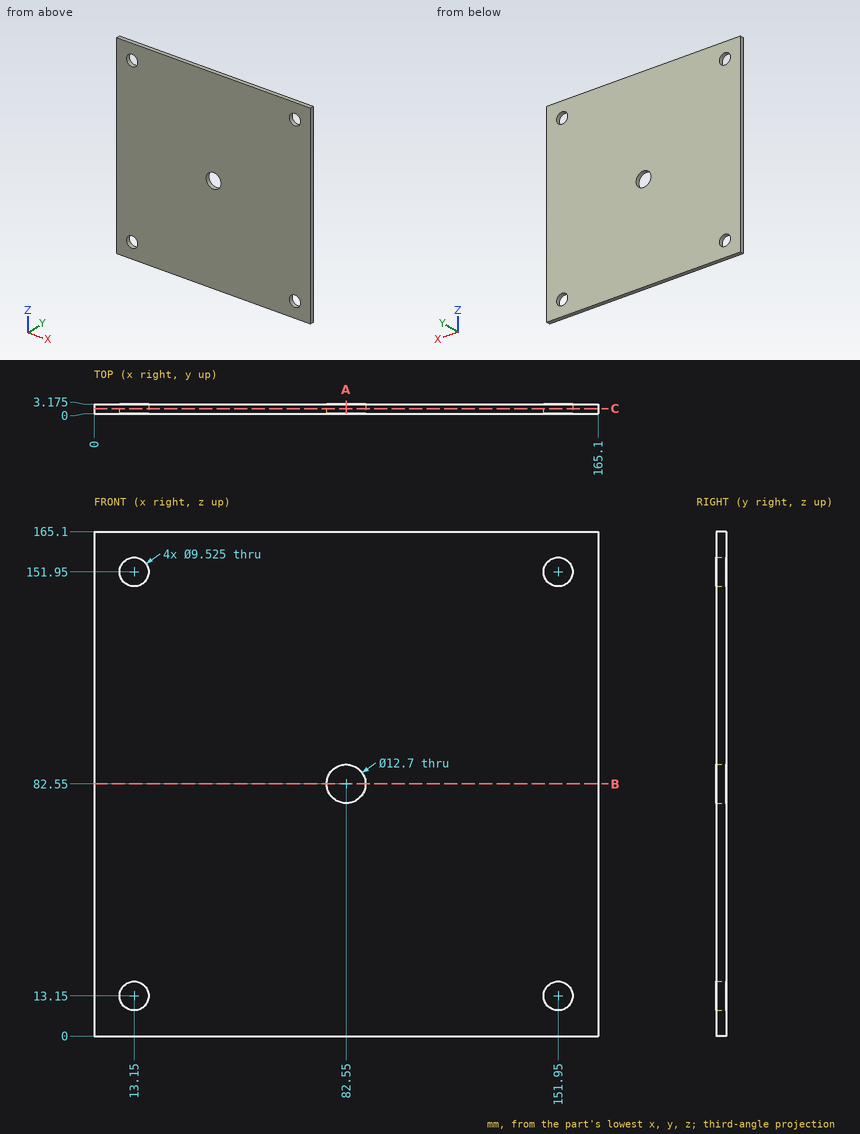
Job drawing, mm, ordinate dimensions from the low corner. One solid piece. Round coordinates to 2 decimals unless told otherwise and drop trailing zeros. Loops run counter-clockwise (first coordinate to the right, second up) from the corner with the lowest first, then second, coordinate; pieces in that order, holes last. Notation, with made-up numbers: (82.5, 46.25) -> (114.5, 46.25) arc R11 cw to (114.5, 53.25) -> close; hole circle Ø4 at (-13, 85). An arc over 180 degrees is marked (long way). Use a Markdown table: item, result.
1) Probe line 1 (Z direction, x = 152.5, y = 1.8); line 2 (Z direction, x = 82.55, y = 1); line 3 (X direction, y = 2.5, z = 15). List the from-to ranges inside material, lowest first. Write a range as [from, to].
The answers:
| item | result |
|---|---|
| line 1 | z = [0, 8.42], [17.88, 147.22], [156.68, 165.1] |
| line 2 | z = [0, 76.2], [88.9, 165.1] |
| line 3 | x = [0, 8.76], [17.54, 147.56], [156.34, 165.1] |
2) Cut at C-C, the plane y = 1.7. State how many separate pieces and enclosed holes the cut face has, and give its area (3 significant figures).
The answers:
| item | result |
|---|---|
| separate pieces | 1 |
| enclosed holes | 5 |
| area | 26,800 mm2 |
3) Cut at B-B, the plane z = 82.55. List the corners of the cut face in (x, y) (1 decimal), and give its area (3 significant figures).
The answers:
| item | result |
|---|---|
| outline | (0, 0) -> (76.2, 0) -> (76.2, 3.2) -> (0, 3.2) -> close; (88.9, 0) -> (165.1, 0) -> (165.1, 3.2) -> (88.9, 3.2) -> close |
| area | 484 mm2 |
4) Cut at A-A, the plane x = 82.55. List the corners of the cut face in (y, z) (1 decimal), and give its area (3 significant figures).
The answers:
| item | result |
|---|---|
| outline | (0, 0) -> (3.2, 0) -> (3.2, 76.2) -> (0, 76.2) -> close; (0, 88.9) -> (3.2, 88.9) -> (3.2, 165.1) -> (0, 165.1) -> close |
| area | 484 mm2 |
